Source: three-view drawing plus pictorial views. Frame: mm from the lowest corner of the part. Give positions to 0.01 mm unless a question says otherwise; leave off trailing zeros. Order: outer loops, then holes, each group sorted by start corner. A loop starts at its lowest first (then second) coordinate and runs counter-clockwise, first axis right, second up. Notation, with made-up numbers: (-30, 76.5) -> (0, 76.5) arc R8 cw to (0, 81.5) -> close; hole circle Ø7 at (8, 81.5). An arc over 180 degrees is marked (long way). One line per question, with ' | ' between items.
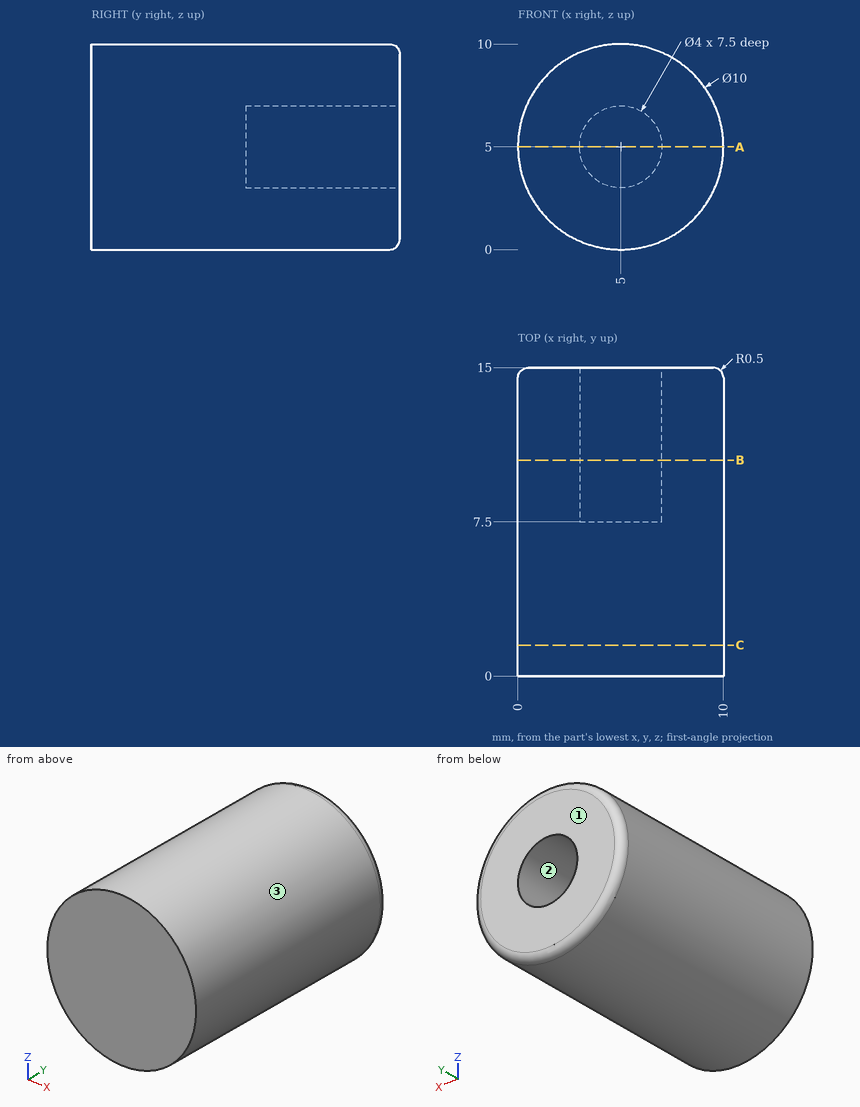
1) Contact query for flat-ended pins moving along their axis: pin 1 Ø3 at (y, z) = (7.5, 6.5) entering from -X; pin 2 Ø1 at (y, z) = (12.5, 8) entering from +X; pin 3 Ø6 at (x, y) = (9, 2) entering from -Z; pin 4 Ø1.5 at (y, z) = (10.5, 7.5) entering from +X. Output: stop coordinate, or through.
Check result:
pin 1: stops at x = 0 | pin 2: stops at x = 9.33 | pin 3: stops at z = 0.1 | pin 4: stops at x = 9.68
2) Section B-B on y = 10.5. Return loops of the section in (x, z).
Check result:
outline: circle Ø10 at (5, 5); hole circle Ø4 at (5, 5)
3) Pull-direction query (Z, two-part tool) for the marked faces 1, 2 and 3; classes: +Z half, -Z half, draft (parallel to the pull), parting line (faces both ways), or undercut.
Check result:
face 1: draft | face 2: undercut | face 3: parting line
4) Section A-A on z = 5. Return loops of the section in (x, y).
Check result:
outline: (0, 0) -> (10, 0) -> (10, 14.5) arc R0.5 ccw to (9.5, 15) -> (7, 15) -> (7, 7.5) -> (3, 7.5) -> (3, 15) -> (0.5, 15) arc R0.5 ccw to (0, 14.5) -> close
5) Material intervals for probe 1 along Z at (x, y) = (5, 12.25); probe 2 along Z at (x, y) = (4.5, 9.25); probe 3 along X at (y, z) = (9.25, 3.75), sorted ascending. Write a range as from..to.
Check result:
probe 1: z = 0..3, 7..10 | probe 2: z = 0.03..3.06, 6.94..9.97 | probe 3: x = 0.16..3.44, 6.56..9.84
6) Section C-C on y = 1.5. Return loops of the section in (x, z).
Check result:
outline: circle Ø10 at (5, 5)
